from build123d import *

# Parameters (mm, degrees)
SKETCH1_W             = 5.9
SKETCH1_H             = 5.8
BOSS_EXTRUDE1_DEPTH   = 4
BOSS_EXTRUDE2_DEPTH   = 5.8
FILLET1_R             = 2
M2X0_4_TAPPED_HOLE1_D = 1.6


with BuildPart() as part:
    # Sketch1 → Boss-Extrude1 (new body)
    with BuildSketch(Plane(origin=(0, 0, 0), x_dir=(1, 0, 0), z_dir=(0, 1, 0))):
        with Locations((-8.45, 0)):
            Rectangle(SKETCH1_W, SKETCH1_H)
    extrude(amount=BOSS_EXTRUDE1_DEPTH)

    # Sketch2 → Boss-Extrude2 (add)
    with BuildSketch(Plane.XY.offset(2.9)):
        with BuildLine():
            Line((-10.5, 0), (-5.5, 0))
            ThreePointArc((-5.5, 0), (0, 5.5), (5.5, 0))
            Line((5.5, 0), (10.5, 0))
            ThreePointArc((10.5, 0), (0, 10.5), (-10.5, 0))
        make_face()
    extrude(amount=-BOSS_EXTRUDE2_DEPTH)


with BuildPart() as body_2:
    # Mirror3: mirrored copy
    add(part.part.mirror(Plane(origin=(0, 0, 0), x_dir=(0, 0, 1), z_dir=(1, 0, 0))))


with BuildPart() as part_1:
    add(part.part)

    # Combine1: union body 2
    add(body_2.part)

    # Fillet1
    fillet1_edges = [part_1.edges().sort_by_distance(p)[0] for p in [
        (-11.4, 2, -2.9),
        (-11.4, 2, 2.9),
        (11.4, 2, -2.9),
        (11.4, 2, 2.9),
    ]]
    fillet(fillet1_edges, radius=FILLET1_R)

    # M2x0.4 Tapped Hole1 (through all)
    with Locations(Plane(origin=(0, 0, 0), x_dir=(-1, 0, 0), z_dir=(0, -1, 0))):
        with Locations((-8.5, 0), (8.5, 0)):
            Hole(M2X0_4_TAPPED_HOLE1_D / 2)


solid = part_1.part
Here's how the part is built. I have some questions about the finished solid (model axes, mm). A direction names the side the tool comes from. Coordinates: 2 decimals unless noted, no trailing zeros. Order: outer loops, then holes, each group sorted by start corner. A loop starts at its lowest first (then second) coordinate and runs counter-clockwise, first axis right, second up.
Item 1: If we section it at B-B on z = -0.35: List the corners of the cut face in (x, y) for me.
Result sheet:
outline: (-11.4, 0) - (-9.22, 0) - (-9.22, 5.03) arc R10.5 ccw to (-9.71, 4) - (-11.4, 4) - close; (-7.78, 0) - (-5.5, 0) arc R5.5 cw to (5.5, 0) - (7.78, 0) - (7.78, 7.05) arc R10.5 ccw to (-7.78, 7.05) - close; (9.22, 0) - (11.4, 0) - (11.4, 4) - (9.71, 4) arc R10.5 ccw to (9.22, 5.03) - close
Item 2: If we section it at C-C on x = 8.5: List the corners of the cut face in (y, z) for me, plus the area to 3 significant figures.
Result sheet:
outline: (0, -2.9) - (6.16, -2.9) - (6.16, -0.8) - (0, -0.8) - close; (0, 0.8) - (6.16, 0.8) - (6.16, 2.9) - (0, 2.9) - close
area: 25.9 mm2
Item 3: If we section it at A-A on y = 2.5: List the corners of the cut face in (x, z) for me.
Result sheet:
outline: (-11.4, -0.9) arc R2 ccw to (-9.4, -2.9) - (-4.9, -2.9) - (-4.9, 2.9) - (-9.4, 2.9) arc R2 ccw to (-11.4, 0.9) - close; (4.9, -2.9) - (9.4, -2.9) arc R2 ccw to (11.4, -0.9) - (11.4, 0.9) arc R2 ccw to (9.4, 2.9) - (4.9, 2.9) - close; hole circle Ø1.6 at (-8.5, 0); hole circle Ø1.6 at (8.5, 0)
Item 4: If we mould it in two halves opening along X, with no side actions, what happens to faces 1 (the face through (7.7, 2.8, 0)), 2 (the face through (0.2, 10.5, 0)), 3 (the face through (11, 4, 0))? For each: +X half, -X half, draft (parallel to the pull), parting line (faces both ways), or undercut.
Result sheet:
face 1: undercut
face 2: parting line
face 3: draft
Item 5: I need wall thicknesses on line 1 (Z direction, x = 8.5, y = 5.75); line 2 (Y direction, x = -10, z = 2.3); line 3 (X direction, y = 5, z = -1.25). Which ranges of each line are inside material? Lowest first, please.
Result sheet:
line 1: z = -2.9 to -0.8, 0.8 to 2.9
line 2: y = 0 to 4
line 3: x = -9.23 to -2.29, 2.29 to 9.23
Item 6: For P1, Ø1.4, axis at x = -10.5, z = 0, coming from the +Y side; P2, Ø3, axis at y = 7.5, z = 1.5, coming from the +X side; P3, Ø1.5, axis at y = 7, z = 1, coming from the -X side, each with a flat end and sliding along its axis, tell me the tip position at first contact or that it passes through.
Result sheet:
P1: stops at y = 4
P2: stops at x = 8.62
P3: stops at x = -8.44
Item 7: If we section it at D-D on z = 2.5: List the corners of the cut face in (x, y) for me.
Result sheet:
outline: (-10.6, 0) - (-5.5, 0) arc R5.5 cw to (5.5, 0) - (10.6, 0) - (10.6, 4) - (9.71, 4) arc R10.5 ccw to (-9.71, 4) - (-10.6, 4) - close
Item 8: For faces 4 (the face through (0, 6, 2.9)), 5 (the face through (-11, 4, 0)), which set-ups out of +Z, -Z, +X, -X, +Y, -Y let a thin tool reach every point of the face, with its end or its side?
Result sheet:
face 4: +Z, +X, -X, +Y, -Y
face 5: +Z, -Z, -X, +Y
